Check sheet for the modelled part. Datum: model origin and axes. Units: mm. A direction names the side the tool comes from. Round coordinates to 2 decimals unless told otherwise and drop trailing zeros. Loops run counter-clockwise (first coordinate to the right, second up) from the corner with the lowest first, then second, coordinate; pieces in that order, holes last. Notation, with made-up numbers: (74, -10.5) -> (129, -10.5) arc R10 cw to (129, 7.5) -> close; hole circle Ø2 at (16, 44.5). An arc over 180 degrees is marked (long way). One line per item, written item: value. Start each with the question number.
1. Cross-section at C-C on y = -65.5. Record the cut outline in (x, z), then the cut area to 3 significant figures.
2. Set-up check for faces 1 (the face through (2, 0, 6)), 2 (the face through (4.5, -70, 0)), 3 (the face through (0, -70, -4.5)): record each of +Z, -Z, +X, -X, +Y, -Y from which the full face is reachable in a straight line by a thin tool's end or side.
3. Cross-section at B-B on x = 0. Record the cut outline in (y, z).
4. Material ranges on L1, parallel to Y at x = 5.5, z = -2.75; L2, parallel to Y at x = -1, z = -5.25; L3, parallel to X at y = -48.5, z = -4.5, recorded low to high.
5. Cross-section at A-A on z = 0. Record the cut outline in (x, y), then the cut area to 3 significant figures.
6. Go/stop test with flat-tipped pins: pin 1 (6 mm diameter, centred on x = -3.5, y = -57, fed in from +Z); pin 2 (8 mm diameter, centred on y = -3.5, z = 3, fed in from +X); pin 3 (4 mm diameter, centred on y = -32, z = 0, fed in from -X). Record where each tip stops, or that it passes through.
7. Cross-section at D-D on y = -47. Record the cut outline in (x, z), then the cut area to 3 significant figures.
from build123d import *

# Parameters (mm, degrees)
F0_R     = 6
F1_DEPTH = 75
F3_DEPTH = 11
F4_R     = 8
F5_DEPTH = 26
F6_SIZE2 = 0.4374433176
F6_SIZE  = 5


with BuildPart() as f1:
    # F0 (on Front) → F1 (new body)
    with BuildSketch(Plane.XZ):
        Circle(F0_R)
    extrude(amount=F1_DEPTH)

    # F2 (on face) → F3 (cut)
    with BuildSketch(Plane.XZ.offset(75)):
        with BuildLine():
            Line((4.5, 3.9686269666), (4.5, -3.9686269666))
            ThreePointArc((4.5, -3.9686269666), (5.6124860802, -2.1213203436), (6, 0))
            ThreePointArc((6, 0), (5.6124860802, 2.1213203436), (4.5, 3.9686269666))
        make_face()
        with BuildLine():
            ThreePointArc((3.9686269666, 4.5), (0, 6), (-3.9686269666, 4.5))
            Line((-3.9686269666, 4.5), (3.9686269666, 4.5))
        make_face()
        with BuildLine():
            Line((3.9686269666, -4.5), (-3.9686269666, -4.5))
            ThreePointArc((-3.9686269666, -4.5), (0, -6), (3.9686269666, -4.5))
        make_face()
        with BuildLine():
            ThreePointArc((-4.5, 3.9686269666), (-6, 0), (-4.5, -3.9686269666))
            Line((-4.5, -3.9686269666), (-4.5, 3.9686269666))
        make_face()
    extrude(amount=-F3_DEPTH, mode=Mode.SUBTRACT)

    # F4 (on face) → F5 (join)
    with BuildSketch(Plane(origin=(0, 0, 0), x_dir=(-1, 0, 0), z_dir=(0, 1, 0))):
        Circle(F4_R)
    extrude(amount=F5_DEPTH)

    # F6
    f6_edges = [f1.edges().sort_by_distance(p)[0] for p in [
        (8, 26, 0),
    ]]
    f6_side = f1.faces().sort_by_distance((8, 13, 0))[0]
    chamfer(f6_edges, length=F6_SIZE, length2=F6_SIZE2, reference=f6_side)


solid = f1.part
Taken from the geometry:
1. outline: (-4.5, -3.97) arc R6 ccw to (-3.97, -4.5) -> (3.97, -4.5) arc R6 ccw to (4.5, -3.97) -> (4.5, 3.97) arc R6 ccw to (3.97, 4.5) -> (-3.97, 4.5) arc R6 ccw to (-4.5, 3.97) -> close
1. area: 80.5 mm2
2. face 1: -Y
2. face 2: +Z, -Z, +X, -Y
2. face 3: -Z, +X, -X, -Y
3. outline: (-75, -4.5) -> (-64, -4.5) -> (-64, -6) -> (0, -6) -> (0, -8) -> (21, -8) -> (26, -7.56) -> (26, 7.56) -> (21, 8) -> (0, 8) -> (0, 6) -> (-64, 6) -> (-64, 4.5) -> (-75, 4.5) -> close
4. L1: y = 0 to 26
4. L2: y = -64 to 26
4. L3: x = -3.97 to 3.97
5. outline: (-8, 0) -> (-6, 0) -> (-6, -64) -> (-4.5, -64) -> (-4.5, -75) -> (4.5, -75) -> (4.5, -64) -> (6, -64) -> (6, 0) -> (8, 0) -> (8, 21) -> (7.56, 26) -> (-7.56, 26) -> (-8, 21) -> close
5. area: 1,280 mm2
6. pin 1: stops at z = 5.98
6. pin 2: stops at x = 7.93
6. pin 3: stops at x = -6
7. outline: circle Ø12 at (0, 0)
7. area: 113 mm2
